```python
from build123d import *

# Parameters (mm, degrees)
F0_R     = 18.5
F1_DEPTH = 25


with BuildPart() as f1:
    # F0 (on Top) → F1 (new body)
    with BuildSketch(Plane.XY):
        Polygon((19.918584, 34.5), (-19.918584, 34.5), (-39.837169, 0), (-19.918584, -34.5), (19.918584, -34.5), (39.837169, 0), align=None)
        Circle(F0_R, mode=Mode.SUBTRACT)
    extrude(amount=F1_DEPTH)

    # F2 (on Front) → F3 (revolve, cut)
    with BuildSketch(Plane.XZ):
        with BuildLine():
            Line((-48.746884, 0), (-39.837169, 0))
            Line((-39.837169, 0), (-39.837169, 15))
            ThreePointArc((-39.837169, 15), (-36.908236, 22.071068), (-29.837169, 25))
            Line((-29.837169, 25), (0.146632, 25))
            Line((0.146632, 25), (0.146632, 38.46572))
            Line((0.146632, 38.46572), (-48.746884, 38.46572))
            Line((-48.746884, 38.46572), (-48.746884, 0))
        make_face()
    revolve(axis=Axis((0.146632, 0, 31.73286), (0, 0, 1)), mode=Mode.SUBTRACT)


solid = f1.part
```
Could you check a few things on this model? Use its own coordinates, in mm. Coordinates: 2 decimals unless noted, no trailing zeros. Order: outer loops, then holes, each group sorted by start corner. A loop starts at its lowest first (then second) coordinate and runs counter-clockwise, first axis right, second up. Notation, with made-up numbers: M -31.75,9 L 10.25,9 A22 cw 10.25,40 Z; hole C -16.5,82 d8. An arc over 180 degrees is marked long. Use one line per item in the form item = value. Start each with the question number.
1. Suppose I cut it at A-A on z = 11.25. Write out the boundary of the cut face in (x, y), then the cut area to 3 significant figures.
2. Suppose I cut it at B-B on z = 21.75. Write out the boundary of the cut face in (x, y), then the cut area to 3 significant figures.
3. Please list where these lines run through material, in increasing order: line 1 (Y direction, x = 0, z = 7); line 2 (Z direction, x = -25.5, y = -16.5); line 3 (Y direction, x = -8, z = 19).
4. For pin 1 (2 mm diameter, centred on x = 29.5, z = 11, fed in from +Y); pin 2 (2 mm diameter, centred on y = 19.5, z = 6, fed in from +X), each with a flat end and sliding along its axis, tell me the tip position at first contact or that it passes through.
5. We'd pull the mould along X, two halves only. Please class faces 1 (the cylindrical face through (-4.01, -18.06, 12.32)), 2 (the flat face through (29.74, -17.49, 11.82)), 3 (the flat face through (-30.017, -17.009, 11.762)), 4 (the flat face through (-14, -13, 25)): +X half, -X half, draft (parallel to the pull), parting line (faces both ways), or undercut.
Geometry says:
q1.outline = M -39.84,0 L -19.92,-34.5 L 19.92,-34.5 L 39.84,0 L 19.92,34.5 L -19.92,34.5 Z; hole C 0,0 d37
q1.area = 3,050 mm^2
q2.outline = M -36.86,-5.16 L -22.83,-29.47 A37.36 ccw -14.19,-34.5 L 14.49,-34.5 A37.36 ccw 22.59,-29.87 L 37.24,-4.51 A37.36 ccw 37.24,4.51 L 22.59,29.87 A37.36 ccw 14.49,34.5 L -14.19,34.5 A37.36 ccw -22.83,29.47 L -36.86,5.16 A37.36 ccw Z; hole C 0,0 d37
q2.area = 2,980 mm^2
q3.line_1 = -34.5 to -18.5, 18.5 to 34.5
q3.line_2 = 0 to 24.99
q3.line_3 = -34.5 to -16.68, 16.68 to 34.5
q4.pin_1 = 19.64
q4.pin_2 = 29.16
q5.face_1 = undercut
q5.face_2 = +X half
q5.face_3 = -X half
q5.face_4 = draft
